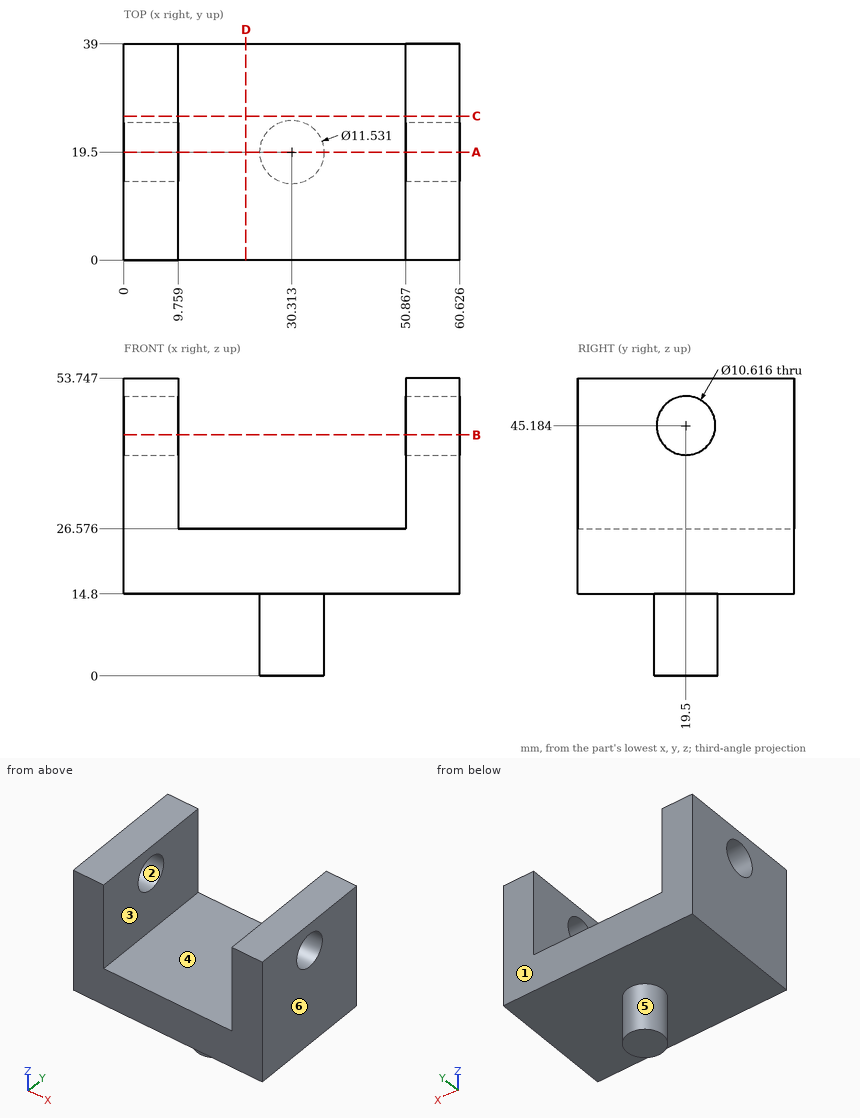
Part print with two shaded views. Sizes in mm from the minimum x, y, z corner. A direction names the side the tool comes from. Round coordinates to 2 decimals unless told otherwise and drop trailing zeros. Write each loop counter-clockwise with the first axis right and the second up, starting at its lowest first coordinate (ties: lowest second). Pieces come first, ordered by that corner, then holes. Notation, with made-up numbers: (-10, -19) -> (12, -19) arc R12 cw to (12, 4) -> close; hole circle Ø3 at (65, 36). An arc over 180 degrees is marked (long way). Put each result on its own line as item: value.
Item 1: Flat gauge pins, fed straight in: P1, Ø8, axis at y = 6, z = 20, coming from the -X side; P2, Ø10, axis at x = 7.5, y = 19, coming from the -Z side; P3, Ø8, axis at x = 44.5, y = 21.5, coming from the +Z side. Where does each tip first touch, or does it go through?
Here are the results:
P1: stops at x = 0
P2: stops at z = 14.8
P3: stops at z = 26.58
Item 2: Slice it at C-C, the plane y = 26. Give the cut face in (x, z), plus the area to 3 significant figures.
Here are the results:
outline: (0, 14.8) -> (60.63, 14.8) -> (60.63, 53.75) -> (50.87, 53.75) -> (50.87, 26.58) -> (9.76, 26.58) -> (9.76, 53.75) -> (0, 53.75) -> close
area: 1,240 mm^2
Item 3: Wall check: probe 1 along Z at (x, y) = (7.75, 19.5) (1 decimal); probe 2 along X at (y, z) = (13.5, 50); probe 3 along Z at (x, y) = (29.5, 29). Give the ranges that are in metal, low to high. Write a range as from..to.
Here are the results:
probe 1: z = 14.8..39.9, 50.5..53.7
probe 2: x = 0..9.76, 50.87..60.63
probe 3: z = 14.8..26.58
Item 4: Slice it at D-D, the plane x = 22. Give the cut face in (y, z).
Here are the results:
outline: (0, 14.8) -> (39, 14.8) -> (39, 26.58) -> (0, 26.58) -> close
Item 5: Two-plate mould, pull along Y, no slides. Class the marked faces 1, 2 and 3: pulls with the +Y half, pulls with the -Y half, needs draft (parallel to the pull), parting line crosses it, or undercut.
Here are the results:
face 1: pulls with the +Y half
face 2: undercut
face 3: needs draft
Item 6: Tool access for the marked faces 4, 5 and 6: list every direction of +Z, -Z, +X, -X, +Y, -Y with a clear straight run to the whole face (end or side of a thin tool).
Here are the results:
face 4: +Z, +Y, -Y
face 5: -Z
face 6: +Z, -Z, +X, +Y, -Y
Item 7: Slice it at A-A, the plane y = 19.5. Give the cut face in (x, z) (1 decimal), plus the area to 3 significant figures.
Here are the results:
outline: (0, 14.8) -> (24.5, 14.8) -> (24.5, 0) -> (36.1, 0) -> (36.1, 14.8) -> (60.6, 14.8) -> (60.6, 39.9) -> (50.9, 39.9) -> (50.9, 26.6) -> (9.8, 26.6) -> (9.8, 39.9) -> (0, 39.9) -> close; (0, 50.5) -> (9.8, 50.5) -> (9.8, 53.7) -> (0, 53.7) -> close; (50.9, 50.5) -> (60.6, 50.5) -> (60.6, 53.7) -> (50.9, 53.7) -> close
area: 1,210 mm^2
Item 8: Slice it at B-B, the plane z = 43.5. Give the cut face in (x, y).
Here are the results:
outline: (0, 0) -> (9.76, 0) -> (9.76, 14.47) -> (0, 14.47) -> close; (0, 24.53) -> (9.76, 24.53) -> (9.76, 39) -> (0, 39) -> close; (50.87, 0) -> (60.63, 0) -> (60.63, 14.47) -> (50.87, 14.47) -> close; (50.87, 24.53) -> (60.63, 24.53) -> (60.63, 39) -> (50.87, 39) -> close
